Verification items for the finished model (mm, model axes). A direction names the side the tool comes from. Coordinates: 2 decimals unless noted, no trailing zeros. Write each loop counter-clockwise with the first axis right and the second up, starting at its lowest first coordinate (ties: lowest second). Pieces come first, ordered by that corner, then holes. Notation, with made-up numbers: M 15.5,31 L 33.5,31 A20 cw 33.5,59 Z; hole C 88.5,13.5 d3. An arc over 180 degrees is marked long. One line per item, written item: value.
```python
from build123d import *

# Parameters (mm, degrees)
F0_W     = 4
F0_H     = 21
F1_DEPTH = 4
F2_R     = 1
F3_W     = 73
F3_H     = 2
F4_DEPTH = 2
F5_R     = 1


with BuildPart() as f1:
    # F0 (on Top) → F1 (new body)
    with BuildSketch(Plane.XY):
        Polygon((0, 25), (0, 0), (73, 0), (73, 25), (68, 25), align=None)
        with Locations((6, 12.5)):
            Rectangle(F0_W, F0_H, mode=Mode.SUBTRACT)
        with Locations((14, 12.5)):
            Rectangle(F0_W, F0_H, mode=Mode.SUBTRACT)
        with Locations((22, 12.5)):
            Rectangle(F0_W, F0_H, mode=Mode.SUBTRACT)
        with Locations((30, 12.5)):
            Rectangle(F0_W, F0_H, mode=Mode.SUBTRACT)
        with Locations((38, 12.5)):
            Rectangle(F0_W, F0_H, mode=Mode.SUBTRACT)
        with Locations((46, 12.5)):
            Rectangle(F0_W, F0_H, mode=Mode.SUBTRACT)
        with Locations((54, 12.5)):
            Rectangle(F0_W, F0_H, mode=Mode.SUBTRACT)
        with Locations((62, 12.5)):
            Rectangle(F0_W, F0_H, mode=Mode.SUBTRACT)
        with Locations((70, 12.5)):
            Rectangle(F0_W, F0_H, mode=Mode.SUBTRACT)
    extrude(amount=F1_DEPTH)

    # F2
    f2_edges = [f1.edges().sort_by_distance(p)[0] for p in [
        (8, 12.5, 4),
        (12, 12.5, 4),
        (16, 12.5, 4),
        (20, 12.5, 4),
        (24, 12.5, 4),
        (28, 12.5, 4),
        (32, 12.5, 4),
        (36, 12.5, 4),
        (40, 12.5, 4),
        (44, 12.5, 4),
        (48, 12.5, 4),
        (52, 12.5, 4),
        (56, 12.5, 4),
        (60, 12.5, 4),
        (64, 12.5, 4),
        (68, 12.5, 4),
    ]]
    fillet(f2_edges, radius=F2_R)

    # F3 (on face) → F4 (join)
    with BuildSketch(Plane.XY.offset(4)):
        with Locations((36.5, 1)):
            Rectangle(F3_W, F3_H)
        with Locations((36.5, 24)):
            Rectangle(F3_W, F3_H)
    extrude(amount=F4_DEPTH)

    # F5
    f5_edges = [f1.edges().sort_by_distance(p)[0] for p in [
        (4, 12.5, 4),
        (0, 12.5, 4),
    ]]
    fillet(f5_edges, radius=F5_R)


solid = f1.part
```
Item 1: Scan lines: line 1 (Y direction, x = 13, z = 3); line 2 (Z direction, x = 66, y = 13.5). Record each from-to range of solid material in increasing order.
The answers:
line 1: y = 0 to 2, 23 to 25
line 2: z = 0 to 4
Item 2: Draft check along X on faces 6 (the face through (36, 0, 3)), 7 (the face through (73, 12, 2)), 8 (the face through (24, 12, 1)). Enter one of: released by +X, released by -X, zero draft, split by the parting line, or undercut.
The answers:
face 6: zero draft
face 7: released by +X
face 8: undercut
Item 3: Cross-section at A-A, the plane z = 4.85. Enter the section's corners in (x, y), and give its area (3 significant figures).
The answers:
outline: M 0,0 L 73,0 L 73,2 L 0,2 Z; M 0,23 L 73,23 L 73,25 L 0,25 Z
area: 292 mm²
Item 4: Cross-section at C-C, the plane y = 7.25. Give the number of separate pieces and of enclosed holes in the cut face, and give its area (3 significant figures).
The answers:
separate pieces: 10
enclosed holes: 0
area: 144 mm²
Item 5: Cross-section at B-B, the plane x = 14. Enter the section's corners in (y, z).
The answers:
outline: M 0,0 L 2,0 L 2,6 L 0,6 Z; M 23,0 L 25,0 L 25,6 L 23,6 Z
Item 6: Access from +Z, -Z, +X, -X, +Y, -Y to the whole of each face (thin tool, end or side, straight path). Record for faces 1 (the face through (36, 24, 6)), 2 (the face through (50, 13, 4)), 3 (the face through (44, 23, 4)), 4 (the face through (37, 25, 3)), 5 (the face through (56, 12, 1)).
The answers:
face 1: +Z, +X, -X, +Y, -Y
face 2: +Z, +X, -X
face 3: +Z
face 4: +Z, -Z, +X, -X, +Y
face 5: +Z, -Z
Item 7: Go/stop test with a flat-tipped pin: P1, Ø1, axis at x = 50, y = 11.5, coming from the +Z side. Record where the tip stops, or that it passes through.
The answers:
P1: stops at z = 4
